Can you work these out from the model? Positions are in its coordinate system, mm. A direction names the side the tool comes from. Give positions to 0.01 mm unless a question says otherwise; leave off trailing zeros. Order: outer loops, then holes, each group sorted by start corner. A loop starts at its lowest first (then second) coordinate and runs counter-clockwise, first axis right, second up. Notation, with made-up numbers: M 23,57 L 52,57 A6 cw 52,63 Z; hole C 64,-23 d1. An arc over 180 degrees is marked long. Write each question's results on one line, items separated by ' | '.
from build123d import *

# Parameters (mm, degrees)
SKETCH1_R           = 11
SKETCH1_R_2         = 4
BOSS_EXTRUDE1_DEPTH = 3.5
CUT_EXTRUDE1_START  = -3.5
SKETCH1_3_R         = 9
SKETCH1_3_R_2       = 6
CUT_EXTRUDE1_DEPTH  = 0.5
CUT_EXTRUDE2_START  = 3
SKETCH1_4_R         = 9
SKETCH1_4_R_2       = 6
CUT_EXTRUDE2_DEPTH  = 0.5
CHAMFER1_SIZE       = 0.5


with BuildPart() as part:
    # Sketch1 → Boss-Extrude1 (new, symmetric)
    with BuildSketch(Plane.XY):
        Circle(SKETCH1_R)
        Circle(SKETCH1_R_2, mode=Mode.SUBTRACT)
    extrude(amount=BOSS_EXTRUDE1_DEPTH, both=True)

    # Sketch1<3> → Cut-Extrude1 (cut)
    with BuildSketch(Plane.XY.offset(CUT_EXTRUDE1_START)):
        Circle(SKETCH1_3_R)
        Circle(SKETCH1_3_R_2, mode=Mode.SUBTRACT)
    extrude(amount=CUT_EXTRUDE1_DEPTH, mode=Mode.SUBTRACT)

    # Sketch1<4> → Cut-Extrude2 (cut)
    with BuildSketch(Plane.XY.offset(CUT_EXTRUDE2_START)):
        Circle(SKETCH1_4_R)
        Circle(SKETCH1_4_R_2, mode=Mode.SUBTRACT)
    extrude(amount=CUT_EXTRUDE2_DEPTH, mode=Mode.SUBTRACT)

    # Chamfer1
    chamfer1_edges = [part.edges().sort_by_distance(p)[0] for p in [
        (-6, 0, -3.5),
        (-9, 0, -3.5),
        (-11, 0, -3.5),
        (-9, 0, 3.5),
        (-6, 0, 3.5),
        (-11, 0, 3.5),
        (-4, 0, -3.5),
        (-4, 0, 3.5),
    ]]
    chamfer(chamfer1_edges, length=CHAMFER1_SIZE - 0.0001)  # a hair under: the kernel refuses the full size


solid = part.part
(1) Will these pins go through, and if not, where does the flat tip stop? P1, Ø2, axis at x = -3, z = -1.5, coming from the +Y side; P2, Ø2, axis at x = 1.5, z = -1, coming from the +Y side; P3, Ø3, axis at y = -3, z = 1.5, coming from the -X side.
Data:
P1: stops at y = 10.82 | P2: stops at y = 10.99 | P3: stops at x = -10.9
(2) I need wall thicknesses on L1, parallel to X at y = 0, z = 3.05; L2, parallel to Y at x = 0, z = -2.95; L3, parallel to Z at x = -7.5, y = 2.5. Which ranges of each line are inside material? Lowest first, please. Write a range as from..to.
Data:
L1: x = -10.95..-9.05, -5.95..-4.05, 4.05..5.95, 9.05..10.95 | L2: y = -11..-4, 4..11 | L3: z = -3..3
(3) Imagine slicing it at A-A, the plane z = 0. Write out the boundary of the cut face in (x, y).
Data:
outline: C 0,0 d22; hole C 0,0 d8
(4) For faces 1 (the face through (-5, -9, -3.5)), 2 (the face through (2, -6, 3)), which set-ups out of +Z, -Z, +X, -X, +Y, -Y let a thin tool reach every point of the face, with its end or its side?
Data:
face 1: -Z, +X, -X, +Y, -Y | face 2: +Z
(5) We'd pull the mould along Y, two halves only. Please class faces 3 (the face through (2, -6, -3)), 4 (the face through (-2.38, -10.74, 0.04)), 5 (the face through (-5, -9, 3.5)), 6 (the face through (-0.867, -3.905, -0.042)): +Y half, -Y half, draft (parallel to the pull), parting line (faces both ways), or undercut.
Data:
face 3: undercut | face 4: parting line | face 5: draft | face 6: undercut
